Part model, mm, in its own coordinate system. Face numbers are marked on the shaded views. A direction names the side the tool comes from. Give positions to 0.01 mm unless a question says otherwise; leave off trailing zeros. Order: outer loops, then holes, each group sorted by start corner. A loop starts at its lowest first (then second) coordinate and runs counter-clockwise, first axis right, second up. Notation, with made-up numbers: (70.5, -5.5) - (76.5, -5.5) arc R19 cw to (76.5, 9.5) - close; hole circle Ø8 at (32, -18). An arc over 180 degrees is marked (long way). One line per item, written item: value.
```python
from build123d import *

# Parameters (mm, degrees)
PAD_DEPTH           = 25
POCKET_DEPTH        = 23.5
PAD001_DEPTH        = 9
SKETCH003_R         = 1.7
POCKET001_DEPTH     = 6
POCKET002_DEPTH     = 5
SKETCH005_W         = 20
SKETCH005_H         = 5.5
POCKET003_DEPTH     = 0.5
SKETCH006_R         = 0.625
SKETCH006_W         = 11
SKETCH006_H         = 6.2
POCKET004_DEPTH     = 5
POCKET005_DEPTH     = 5
POCKET006_DEPTH     = 25.001
LINEARPATTERN_COUNT = 15
LINEARPATTERN_PITCH = 4.285714
POCKET007_DEPTH     = 5


with BuildPart() as part:
    # Sketch → Pad (new body)
    with BuildSketch(Plane.XY):
        with BuildLine():
            Line((-35, 21.5), (35, 21.5))
            ThreePointArc((39.5, 17), (38.181981, 20.181981), (35, 21.5))
            Line((39.5, 17), (39.5, -17))
            ThreePointArc((35, -21.5), (38.181981, -20.181981), (39.5, -17))
            Line((35, -21.5), (-35, -21.5))
            ThreePointArc((-39.5, -17), (-38.181981, -20.181981), (-35, -21.5))
            Line((-39.5, -17), (-39.5, 17))
            ThreePointArc((-35, 21.5), (-38.181981, 20.181981), (-39.5, 17))
        make_face()
    extrude(amount=PAD_DEPTH)

    # Sketch001 (on Face10 of Pad) → Pocket (cut)
    with BuildSketch(Plane.XY.offset(25)):
        with BuildLine():
            Line((35, 20), (-35, 20))
            ThreePointArc((-35, 20), (-37.12132, 19.12132), (-38, 17))
            Line((-38, 17), (-38, -17))
            ThreePointArc((-38, -17), (-37.12132, -19.12132), (-35, -20))
            Line((-35, -20), (35, -20))
            ThreePointArc((35, -20), (37.12132, -19.12132), (38, -17))
            Line((38, -17), (38, 17))
            ThreePointArc((38, 17), (37.12132, 19.12132), (35, 20))
        make_face()
    extrude(amount=-POCKET_DEPTH, mode=Mode.SUBTRACT)

    # Sketch002 (on Face19 of Pocket) → Pad001 (join)
    with BuildSketch(Plane.XY.offset(1.5)):
        with BuildLine():
            Line((-35, 20), (-32.25, 20))
            Line((-32.25, 20), (-32.25, 17.25))
            ThreePointArc((-35.25, 14.25), (-33.12868, 15.12868), (-32.25, 17.25))
            Line((-35.25, 14.25), (-38, 14.25))
            Line((-38, 14.25), (-38, 17))
            ThreePointArc((-35, 20), (-37.12132, 19.12132), (-38, 17))
        make_face()
        with BuildLine():
            Line((35, 20), (32.25, 20))
            Line((32.25, 20), (32.25, 17.25))
            ThreePointArc((32.25, 17.25), (33.12868, 15.12868), (35.25, 14.25))
            Line((35.25, 14.25), (38, 14.25))
            Line((38, 14.25), (38, 17))
            ThreePointArc((38, 17), (37.12132, 19.12132), (35, 20))
        make_face()
        with BuildLine():
            Line((-38, -14.25), (-35.25, -14.25))
            ThreePointArc((-32.25, -17.25), (-33.12868, -15.12868), (-35.25, -14.25))
            Line((-32.25, -17.25), (-32.25, -20))
            Line((-32.25, -20), (-35, -20))
            ThreePointArc((-38, -17), (-37.12132, -19.12132), (-35, -20))
            Line((-38, -17), (-38, -14.25))
        make_face()
        with BuildLine():
            Line((35.25, -14.25), (38, -14.25))
            Line((38, -14.25), (38, -17))
            ThreePointArc((35, -20), (37.12132, -19.12132), (38, -17))
            Line((35, -20), (32.25, -20))
            Line((32.25, -20), (32.25, -17.25))
            ThreePointArc((35.25, -14.25), (33.12868, -15.12868), (32.25, -17.25))
        make_face()
    extrude(amount=PAD001_DEPTH)

    # Sketch003 (on Face19 of Pad001) → Pocket001 (cut)
    with BuildSketch(Plane.XY.offset(10.5)):
        with Locations((-35, 17)):
            Circle(SKETCH003_R)
        with Locations((-35, -17)):
            Circle(SKETCH003_R)
        with Locations((35, -17)):
            Circle(SKETCH003_R)
        with Locations((35, 17)):
            Circle(SKETCH003_R)
    extrude(amount=-POCKET001_DEPTH, mode=Mode.SUBTRACT)

    # Sketch004 (on Face6 of Pocket001) → Pocket002 (cut)
    with BuildSketch(Plane.XZ.offset(21.5)):
        with BuildLine():
            Line((-22, 25), (39.5, 25))
            Line((39.5, 12.1), (39.5, 25))
            Line((-5, 12.1), (39.5, 12.1))
            ThreePointArc((-6.5, 13.6), (-6.06066, 12.53934), (-5, 12.1))
            Line((-6.5, 16), (-6.5, 13.6))
            ThreePointArc((-6.5, 16), (-6.93934, 17.06066), (-8, 17.5))
            Line((-20.5, 17.5), (-8, 17.5))
            ThreePointArc((-22, 19), (-21.56066, 17.93934), (-20.5, 17.5))
            Line((-22, 19), (-22, 25))
        make_face()
    extrude(amount=-POCKET002_DEPTH, mode=Mode.SUBTRACT)

    # Sketch005 (on Face7 of Pocket002) → Pocket003 (cut)
    with BuildSketch(Plane(origin=(0, 21.5, 0), x_dir=(-1, 0, 0), z_dir=(0, 1, 0))):
        with Locations((-21, 19.25)):
            Rectangle(SKETCH005_W, SKETCH005_H)
    extrude(amount=-POCKET003_DEPTH, mode=Mode.SUBTRACT)

    # Sketch006 (on Face7 of Pocket003) → Pocket004 (cut)
    with BuildSketch(Plane(origin=(0, 21.5, 0), x_dir=(-1, 0, 0), z_dir=(0, 1, 0))):
        with Locations((-13.25, 19.425)):
            Circle(SKETCH006_R)
        with Locations((-28.75, 19.075)):
            Circle(SKETCH006_R)
        with Locations((-21, 19.25)):
            Rectangle(SKETCH006_W, SKETCH006_H)
    extrude(amount=-POCKET004_DEPTH, mode=Mode.SUBTRACT)

    # Sketch007 (on Face9 of Pocket004) → Pocket005 (cut)
    with BuildSketch(Plane.YZ.offset(39.5)):
        with BuildLine():
            Line((-11.5, 1.5), (-5.5, 1.5))
            ThreePointArc((-5.5, 1.5), (-4.43934, 1.93934), (-4, 3))
            Line((-4, 3), (-4, 12.1))
            Line((-4, 12.1), (12.75, 12.1))
            ThreePointArc((12.75, 12.1), (13.81066, 12.53934), (14.25, 13.6))
            Line((14.25, 13.6), (14.25, 25))
            Line((14.25, 25), (-16.5, 25))
            Line((-16.5, 12.1), (-16.5, 25))
            Line((-13, 12.1), (-16.5, 12.1))
            Line((-13, 3), (-13, 12.1))
            ThreePointArc((-13, 3), (-12.56066, 1.93934), (-11.5, 1.5))
        make_face()
    extrude(amount=-POCKET005_DEPTH, mode=Mode.SUBTRACT)

    # Sketch008 (on Face4 of Pocket005) → Pocket006 (cut, through all)
    with BuildSketch(Plane(origin=(0, 0, 0), x_dir=(1, 0, 0), z_dir=(0, 0, -1))):
        with BuildLine():
            ThreePointArc((-29, 12.5), (-30, 13.5), (-31, 12.5))
            Line((-31, 12.5), (-31, -12.5))
            ThreePointArc((-31, -12.5), (-30, -13.5), (-29, -12.5))
            Line((-29, -12.5), (-29, 12.5))
        make_face()
    pocket006 = extrude(amount=-POCKET006_DEPTH, mode=Mode.SUBTRACT)

    # LinearPattern: Pocket006 ×15
    with Locations(*[(i * LINEARPATTERN_PITCH, 0, 0) for i in range(1, LINEARPATTERN_COUNT)]):
        add(pocket006, mode=Mode.SUBTRACT)

    # Sketch009 (on Face7 of LinearPattern) → Pocket007 (cut)
    with BuildSketch(Plane(origin=(0, 21.5, 0), x_dir=(-1, 0, 0), z_dir=(0, 1, 0))):
        with BuildLine():
            Line((-5, 25), (29, 25))
            Line((29, 25), (29, 20.925))
            ThreePointArc((27.5, 19.425), (28.56066, 19.86434), (29, 20.925))
            Line((27.5, 19.425), (-3.5, 19.425))
            ThreePointArc((-5, 20.925), (-4.56066, 19.86434), (-3.5, 19.425))
            Line((-5, 20.925), (-5, 25))
        make_face()
    extrude(amount=-POCKET007_DEPTH, mode=Mode.SUBTRACT)


solid = part.part
```
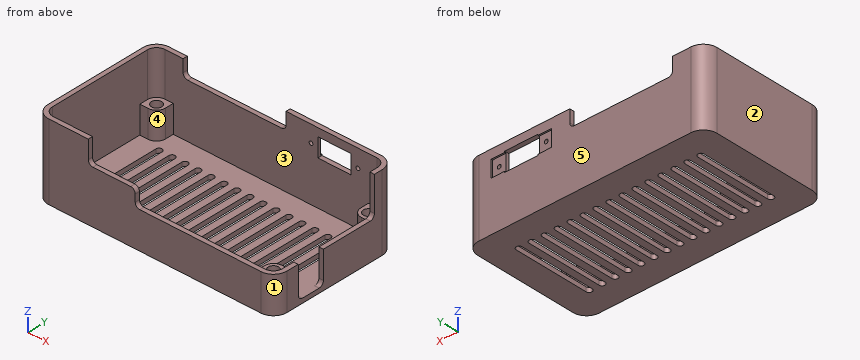
1) Pin check, flat tips, straight feed: pin 1 (4 mm diameter, centred on x = -9, y = 12.5, fed in from +Z); pin 2 (4.5 mm diameter, centred on x = 6.5, y = -18, fed in from +Z); pin 3 (2.5 mm diameter, centred on x = 34.5, y = 17, fed in from +Z). Stop position of each tip, or through.
Outcome:
pin 1: stops at z = 1.5
pin 2: stops at z = 12.1
pin 3: stops at z = 10.5
2) Cut at A-A, the plane z = 15. Give the cut face in (x, y).
Outcome:
outline: (-39.5, -17) arc R4.5 ccw to (-35, -21.5) - (-6.5, -21.5) - (-6.5, -20) - (-35, -20) arc R3 cw to (-38, -17) - (-38, 17) arc R3 cw to (-35, 20) - (35, 20) arc R3 cw to (38, 17) - (38, 14.25) - (39.5, 14.25) - (39.5, 17) arc R4.5 ccw to (35, 21.5) - (-35, 21.5) arc R4.5 ccw to (-39.5, 17) - close
3) Which spindle directions (+Z, -Z, +X, -X, +Y, -Y) get a long thin tool onto all of the face, cutting with end or side? Do the marked faces 4 and 5. Say none if no direction does.
Outcome:
face 4: +Z
face 5: +Z, -Z, +X, -X, +Y
4) Drill centre lines: line 1 along Y through (x, z) = (35, 8.75); line 2 along X through (y, z) = (17, 23.75); line 3 along Z through (x, y) = (13.25, 20.45). Where is each one in solid material? Low to high. Write a range as from..to.
Outcome:
line 1: y = -21.5..-18.7, -15.3..-14.26, 14.26..15.3, 18.7..21.5
line 2: x = -39.5..-38, 38..39.5
line 3: z = 0..18.8, 20.05..25
5) Mould opens along Y. For the marked faces 1, 2 and 3 say: released by +Y, released by -Y, zero draft, split by the parting line, or undercut.
Outcome:
face 1: released by -Y
face 2: zero draft
face 3: undercut
6) Cut at B-B, the plane y = 8.5. Give the number of separate pieces and of enclosed holes in the cut face, then the cut area to 3 significant figures.
Outcome:
separate pieces: 16
enclosed holes: 0
area: 125 mm^2
